```python
from build123d import *

# Parameters (mm, degrees)
F0_R     = 1.5
F1_DEPTH = 141.5
F0_R_2   = 1.3
F2_DEPTH = 141.5
F3_DEPTH = 142.5
F4_DEPTH = 2
F5_R     = 0.99999


# Not quite as in the source:
# - a fillet or chamfer is up to 0.001 mm smaller than in the source, because OpenCascade refuses the exact size


with BuildPart() as f1:
    # F0 (on Front) → F1 (new body)
    with BuildSketch(Plane.XZ):
        with BuildLine():
            Line((0.25, 46.7269286196), (-4.25, 51.2269286196))
            Line((-4.25, 51.2269286196), (-4.25, 3.2269286196))
            ThreePointArc((-4.25, 3.2269286196), (-3.6642135624, 1.8127150573), (-2.25, 1.2269286196))
            Line((-2.25, 1.2269286196), (-1.75, 1.2269286196))
            ThreePointArc((-1.75, 1.2269286196), (-0.3357864376, 1.8127150573), (0.25, 3.2269286196))
            Line((0.25, 3.2269286196), (0.25, 46.7269286196))
        make_face()
        with Locations((-2, 3.4769286196)):
            Circle(F0_R, mode=Mode.SUBTRACT)
    extrude(amount=F1_DEPTH)

    # F0 (on Front) → F2 (join)
    with BuildSketch(Plane.XZ):
        with Locations((-2, 3.4769286196)):
            Circle(F0_R)
        with Locations((-2, 3.4769286196)):
            Circle(F0_R_2, mode=Mode.SUBTRACT)
    extrude(amount=F2_DEPTH)

    # F0 (on Front) → F3 (join)
    with BuildSketch(Plane.XZ):
        with Locations((-2, 3.4769286196)):
            Circle(F0_R_2)
    extrude(amount=F3_DEPTH)

    # F0 (on Front) → F4 (cut)
    with BuildSketch(Plane.XZ):
        with Locations((-2, 3.4769286196)):
            Circle(F0_R)
        with Locations((-2, 3.4769286196)):
            Circle(F0_R_2, mode=Mode.SUBTRACT)
        with Locations((-2, 3.4769286196)):
            Circle(F0_R_2)
    extrude(amount=F4_DEPTH, mode=Mode.SUBTRACT)

    # F5 (radius 1 in the source; OpenCascade refuses exactly that, so slightly less here)
    f5_edges = [f1.edges().sort_by_distance(p)[0] for p in [
        (-3.3, -142.5, 3.476929),
    ]]
    fillet(f5_edges, radius=F5_R)


solid = f1.part
```
Input: part model. Units: mm. Frame: model coordinates. A direction names the side the tool comes from. Round coordinates to 2 decimals unless told otherwise and drop trailing zeros. Write each loop counter-clockwise with the first axis right and the second up, starting at its lowest first coordinate (ties: lowest second). Pieces come first, ordered by that corner, then holes. Notation, with made-up numbers: (-37.75, 55.25) - (16.25, 55.25) arc R24 cw to (16.25, 71.25) - close; hole circle Ø10 at (-33.75, -27.75). An arc over 180 degrees is marked (long way). Write item = value, one per line.
(1) Access query for faces 1 (the cylindrical face through (-0.614, -0.986, 2.902)), 2 (the flat face through (-2, 0, 27)). Directions: +Z, -Z, +X, -X, +Y, -Y. A direction counts if a zero-diameter tool reaches every point of the face in a straight line with its end or side. Return the directions, or none.
Geometry check:
face_1 = +Y
face_2 = +Z, -Z, +X, -X, +Y
(2) Contact query for flat-ended pins moving along their axis: pin 1 Ø1.5 at (x, z) = (-2, 38.5) entering from -Y; pin 2 Ø2.5 at (x, z) = (-2, 3.48) entering from +Y; pin 3 Ø1 at (x, y) = (-1.5, -87.5) entering from +Z. Output: stop coordinate, or through.
Geometry check:
pin_1 = -141.5
pin_2 = -2
pin_3 = 48.98
(3) Pull-direction query (X, two-part tool) for faces 3 (the flat face through (-4.25, -70, 28)), 4 (the flat face through (-2, -2, 3)), 5 (the flat face through (-1.969, -69.76, 48.945)); classes: +X half, -X half, draft (parallel to the pull), parting line (faces both ways), or undercut.
Geometry check:
face_3 = -X half
face_4 = undercut
face_5 = +X half
(4) Section query A-A on y = -25. Output: boundary loops of the cut face in (x, z), then the cut area to 3 significant figures.
Geometry check:
outline = (-4.25, 3.23) arc R2 ccw to (-2.25, 1.23) - (-1.75, 1.23) arc R2 ccw to (0.25, 3.23) - (0.25, 46.73) - (-4.25, 51.23) - close
area = 213 mm^2
(5) Material intervals for probe 1 along Y at (x, z) = (-1.15, 16); probe 2 along Z at (x, y) = (-2, -0.9); probe 3 along X at (y, z) = (-127.5, 47.5), sorted ascending.
Geometry check:
probe_1 = -141.5 to 0
probe_2 = 1.23 to 1.98, 4.98 to 48.98
probe_3 = -4.25 to -0.52
